Can you work these out from the model? Positions are in its coordinate system, mm. A direction names the side the tool comes from. Round coordinates to 2 decimals unless told otherwise and drop trailing zeros. Write each loop counter-clockwise with the first axis right and the second up, starting at its lowest first coordinate (ties: lowest second). Pieces come first, ordered by that corner, then holes. Notation, with made-up numbers: M 31,5 L 42,5 A33 ccw 42,38 Z; hole C 11,16 d4. An arc over 180 degrees is marked long. Answer as a JSON object with one key per item and string values. Group by question number.
1) If we mould it in two halves opening along Z, with no side actions, what happens to faces 1 (the cylindrical face through (-1.38, -6.2, -27.54)), 2 (the cylindrical face through (-11.012, -49.592, 6.394)), 3 (the flat face through (1, 1, -41.275))? For each: +Z half, -Z half, draft (parallel to the pull), parting line (faces both ways), or undercut.
2) I'm going to push flat-ended pins straight in: pin 1 Ø12 at (y, z) = (12.5, -15) entering from -X; pin 2 Ø21 at (x, y) = (-2, 7) entering from +Z; pin 3 Ø12 at (x, z) = (7.5, -22) entering from +Y; pin 4 Ø3 at (y, z) = (-18, -2) entering from -X. Where does each tip first touch, or does it pass through?
3) On a 3-axis mill with a long thin cutter (end or side, diameter ignored), from which of +Z, -Z, +X, -X, +Y, -Y can I reach the whole of each face in a straight line? I mean faces 4 (the cylindrical face through (-37.794, -28.979, 7.915)), 5 (the flat face through (-15.3, 45.4, 9.525)), 6 (the cylindrical face through (-4.68, 4.29, -4.19)), 7 (the cylindrical face through (-30.235, -23.183, -38.056)). Say none if no direction works.
4) Suppose I cut it at A-A, the plane z = -11.5. Write out the boundary of the cut face in (x, y), and give its area (3 significant figures).
5) Please list where these lines run through material, in increasing order: L1, parallel to Y at x = 0, z = 7 (3 decimals); L2, parallel to Z at x = 11, y = 10 (3 decimals); L3, parallel to Z at x = -33, y = -12.5 (3 decimals). Write a range as [from, to].
from build123d import *

# Parameters (mm, degrees)
F2_R = 3.175


# Not quite as in the source:
# - a feature names something its author has since deleted; it is built from what else it names


with BuildPart() as f1:
    # F0 (on Front) → F1 (revolve)
    with BuildSketch(Plane.XZ):
        Polygon((0, 6.35), (0, 0), (6.35, 0), (50.8, 0), (50.8, 9.525), (47.625, 9.525), (47.625, 6.35), align=None)
        Polygon((6.35, -31.75), (0, -31.75), (0, -41.275), (38.1, -41.275), (38.1, -31.75), align=None)
        with BuildLine():
            Line((6.35, 0), (0, 0))
            Line((0, 0), (0, -4.7625))
            ThreePointArc((0, -4.7625), (3.3277085246, -5.2724525596), (6.35, -6.7555067986))
            Line((6.35, -6.7555067986), (6.35, 0))
        make_face()
        with BuildLine():
            ThreePointArc((6.35, -24.9944932014), (3.3277085246, -26.4775474404), (0, -26.9875))
            Line((0, -26.9875), (0, -31.75))
            Line((0, -31.75), (6.35, -31.75))
            Line((6.35, -31.75), (6.35, -24.9944932014))
        make_face()
        with BuildLine():
            ThreePointArc((6.35, -6.7555067986), (3.3277085246, -5.2724525596), (0, -4.7625))
            Line((0, -4.7625), (0, -26.9875))
            ThreePointArc((0, -26.9875), (3.3277085246, -26.4775474404), (6.35, -24.9944932014))
            Line((6.35, -24.9944932014), (6.35, -6.7555067986))
        make_face()
        with BuildLine():
            ThreePointArc((11.1125, -15.875), (9.8501784565, -10.7309120706), (6.35, -6.7555067986))
            Line((6.35, -6.7555067986), (6.35, -24.9944932014))
            ThreePointArc((6.35, -24.9944932014), (9.8501784565, -21.0190879294), (11.1125, -15.875))
        make_face()
    revolve(axis=Axis((0, 0, 19.689680915), (0, 0, 1)))

    # F2
    f2_edges = [f1.edges().sort_by_distance(p)[0] for p in [
        (-6.35, 0, 0),
        (-6.35, 0, -6.755507),
        (11.1125, 0, -15.875),
        (6.35, 0, -3.377753),
        (-6.35, 0, -24.994493),
        (6.35, 0, -28.372247),
        (-6.35, 0, -31.75),
        (-50.8, 0, 0),
        (-38.1, 0, -31.75),
    ]]
    fillet(f2_edges, radius=F2_R)


solid = f1.part
Results:
{
 "1": {"face 1": "undercut", "face 2": "draft", "face 3": "-Z half"},
 "2": {"pin 1": "x = -8.99", "pin 2": "z = 6.35", "pin 3": "y = 10.48", "pin 4": "through"},
 "3": {"face 4": "+Z", "face 5": "+Z, +X, -X, +Y, -Y", "face 6": "none", "face 7": "-Z"},
 "4": {"outline": "C 0,0 d20.43", "area": "328 mm^2"},
 "5": {"L1": "[-50.8, -47.625], [47.625, 50.8]", "L2": "[-41.275, -31.75], [0, 6.35]", "L3": "[-41.275, -31.771], [0, 6.35]"}
}
